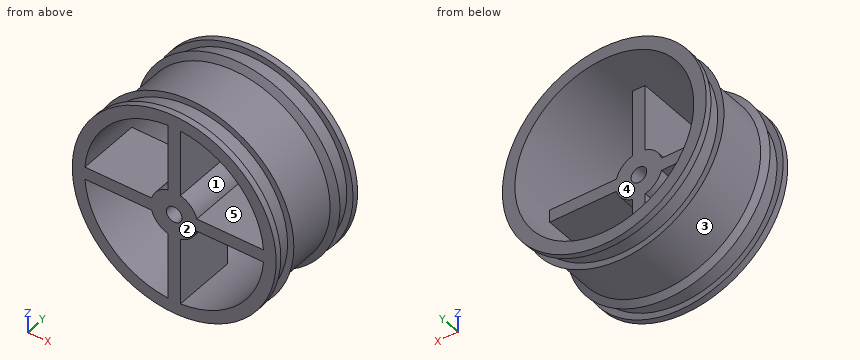
Autodesk Inventor part; units mm, degrees
ref_plane "YZ Plane" through (0, 0, 0) normal (1, 0, 0) x (0, 1, 0)
ref_plane "XZ Plane" through (0, 0, 0) normal (0, 1, 0) x (-1, 0, 0)
ref_plane "XY Plane" through (0, 0, 0) normal (0, 0, 1) x (1, 0, 0)
sketch "Sketch1" plane through (0, 0, 0) normal (0, 0, 1) x (1, 0, 0)
  line L0 (0, 0) -> (30.65, 0)
  line L1 (30.65, 0) -> (30.65, 17.65)
  line L2 (30.65, 0) -> (30.65, 10)
  line L3 (30.65, 17.65) -> (32.65, 17.65)
  line L4 (32.65, 17.65) -> (32.65, 15.65)
  line L5 (32.65, 15.65) -> (30.65, 15.65)
  line L6 (30.65, 10) -> (32.65, 10)
  line L7 (32.65, 10) -> (30.65, 8.4317)
  line L8 (30.65, 0) -> (30.65, -17.65)
  line L9 (30.65, -17.65) -> (32.65, -17.65)
  line L10 (32.65, -17.65) -> (32.65, -15.65)
  line L11 (32.65, -15.65) -> (30.65, -15.65)
  line L12 (30.65, -10) -> (32.65, -10)
  line L13 (30.65, 17.65) -> (28.65, 17.65)
  line L14 (28.65, 17.65) -> (28.65, -17.65)
  line L15 (28.65, -17.65) -> (30.65, -17.65)
  line L16 (32.65, -10) -> (30.65, -8.6227)
  line L17 (0, -24.71) -> (0, 24.71)
  dimension "d1" = 30.65
  dimension "d5" = 10
  dimension "d9" = 2
  dimension "d10" = 2
  dimension "d11" = 2
  dimension "d12" = 2
revolve "Revolution1" add sketch "Sketch1" angle 360 about axis through (0, -10, 0) along (0, 1, 0)
sketch "Sketch2" plane through (0, 17.65, 0) normal (0, 1, 0) x (1, 0, 0)
  circle A0 centre (0, 0) radius 28.65
  circle A1 centre (0, 0) radius 7.5
  circle A2 centre (0, 0) radius 28.65
  line L0 (-7.2284, -2) -> (-28.5801, -2)
  line L1 (-38.7788, 0) -> (46.3448, 0) construction
  line L2 (-7.2284, 2) -> (-28.5801, 2)
  line L3 (-7.2284, -2) -> (-7.2284, 2) construction
  line L4 (-7.2284, 2) -> (-29.2518, 2) construction
  line L5 (-29.2518, 2) -> (-29.2518, -2) construction
  line L6 (-29.2518, -2) -> (-7.2284, -2) construction
  line L7 (-7.2284, -2) -> (-7.2284, 2)
  line L8 (-7.2284, 2) -> (-29.2518, 2)
  line L9 (-29.2518, 2) -> (-29.2518, -2)
  line L10 (-29.2518, -2) -> (-7.2284, -2)
  circle A3 centre (0, 0) radius 2.5
  dimension "d14" = 15
  dimension "d16" = 5
extrude "Extrusion1" add sketch "Sketch2" against normal up to surface (35.3 mm away) contours L2 A1 L0 A0 | A0 L10 L9 L8 | A1 L7 picked at (-14.5272, 0.2224) picked at (-5.6523, 0)
pattern_circular "Circular Pattern1" count 4 over 360 about axis through (0, 17.65, 0) along (0, -1, 0) of "Extrusion1"
sketch "Sketch3" plane through (0, 17.65, 0) normal (0, 1, 0) x (1, 0, 0)
  circle A0 centre (0, 0) radius 2.5
  circle A1 centre (0, 0) radius 28.65
extrude "Extrusion2" cut sketch "Sketch3" against normal blind 15
properties part number "OSV Specific Wheel"
Geometry: final body of the model. Coordinates: model frame, mm. Face numbers are marked on the shaded views. A direction names the side the tool comes from. Coordinates: 2 decimals unless noted, no trailing zeros. Order: outer loops, then holes, each group sorted by start corner. A loop starts at its lowest first (then second) coordinate and runs counter-clockwise, first axis right, second up. Notation, with made-up numbers: (-12, 55) -> (29, 55) arc R28 ccw to (29, 79) -> close; hole circle Ø7 at (27.5, 74). An arc over 180 degrees is marked (long way). Answer in a Markdown table with one row per item.
Item 1: Section B-B on y = -11. Output: boundary loops of the cut face in (x, z), plus the area to 3 significant figures.
Return value:
| item | result |
|---|---|
| outline | circle Ø61.3 at (0, 0); hole (-28.58, -2) arc R28.65 ccw to (-2, -28.58) -> (-2, -7.23) arc R7.5 cw to (-7.23, -2) -> close; hole (-28.58, 2) -> (-7.23, 2) arc R7.5 cw to (-2, 7.23) -> (-2, 28.58) arc R28.65 ccw to start; hole circle Ø5 at (0, 0); hole (2, -28.58) arc R28.65 ccw to (28.58, -2) -> (7.23, -2) arc R7.5 cw to (2, -7.23) -> close; hole (2, 7.23) arc R7.5 cw to (7.23, 2) -> (28.58, 2) arc R28.65 ccw to (2, 28.58) -> close |
| area | 869 mm² |
Item 2: Access query for the marked faces 4 and 5. Directions: +Z, -Z, +X, -X, +Y, -Y. A direction counts if a zero-diameter tool reaches every point of the face in a straight line with its end or side. Return the directions, or none.
Return value:
| item | result |
|---|---|
| face 4 | +Y |
| face 5 | +Y, -Y |
Item 3: Ray query, L1, parallel to Z at x = 0, y = -13; L2, parallel to X at y = -11, z = -4.5. Return the intervals inside material, ascending.
Return value:
| item | result |
|---|---|
| L1 | z = -30.65 to -2.5, 2.5 to 30.65 |
| L2 | x = -30.32 to -28.29, -6 to 6, 28.29 to 30.32 |
Item 4: Section D-D on z = 16.5. State how many separate pieces and enclosed holes the cut face has, plus the area to 3 significant figures.
Return value:
| item | result |
|---|---|
| separate pieces | 3 |
| enclosed holes | 0 |
| area | 277 mm² |
Item 5: Draft query along Z for the marked faces 1, 2 and 3. Return one class per face: released by +Z, released by -Z, zero draft, split by the parting line, or undercut.
Return value:
| item | result |
|---|---|
| face 1 | undercut |
| face 2 | zero draft |
| face 3 | split by the parting line |
Item 6: Contact query for flat-ended pins moving along their axis: P1, Ø10, axis at y = -8.5, z = 17.5, coming from the -X side; P2, Ø1, axis at x = 6.5, y = -13.5, coming from the +Z side; P3, Ø6, axis at y = 13, z = -13, coming from the -X side; P4, Ø4, axis at x = 0, z = 0, coming from the +Y side. Output: stop coordinate, or through.
Return value:
| item | result |
|---|---|
| P1 | stops at x = -30.07 |
| P2 | stops at z = 30.06 |
| P3 | stops at x = -30.52 |
| P4 | passes through |
